Build history of the part. All positions in model axes, mm. A direction names the side the tool comes from. Round coordinates to 2 decimals unless told otherwise and drop trailing zeros. Write each loop counter-clockwise with the first axis right and the second up, starting at its lowest first coordinate (ties: lowest second). Pieces come first, ordered by that corner, then holes. Notation, with made-up numbers: (7.25, 53) -> (52.25, 53) arc R26 cw to (52.25, 67) -> close; hole circle Ø9 at (-15.75, 73.25). An arc over 180 degrees is marked (long way). Return JSON: item names as keys, results as strings.
from build123d import *

# Parameters (mm, degrees)
CUT_EXTRUDE_1_DEPTH = 3
FILLET_1_R          = 1
CHAMFER_1_SIZE      = 0.5


with BuildPart() as part:
    # 草图1 → 旋转1 (revolve)
    with BuildSketch(Plane.XY):
        Polygon((0, 0), (0, 5), (4.5, 5), (4.5, 3), (14.5, 3), (14.5, 2.5), (24.5, 2.5), (24.5, 0), align=None)
    revolve(axis=Axis((0, 0, 0), (1, 0, 0)))

    # 草图2 → 切除-拉伸1 (cut)
    with BuildSketch(Plane.ZY):
        Polygon((0, 1.732050808), (-1.5, 0.866025404), (-1.5, -0.866025404), (0, -1.732050808), (1.5, -0.866025404), (1.5, 0.866025404), align=None)
    extrude(amount=-CUT_EXTRUDE_1_DEPTH, mode=Mode.SUBTRACT)

    # 圆角1
    fillet_1_edges = [part.edges().sort_by_distance(p)[0] for p in [
        (0, -5, 0),
    ]]
    fillet(fillet_1_edges, radius=FILLET_1_R)

    # 倒角1
    chamfer_1_edges = [part.edges().sort_by_distance(p)[0] for p in [
        (24.5, -2.5, 0),
    ]]
    chamfer(chamfer_1_edges, length=CHAMFER_1_SIZE)


solid = part.part
Q1. 3-axis set-ups, long thin cutter, end or side, ignore diameter. For faces 4 (the cylindrical face through (19.32, -0.54, -2.44)), 5 (the flat face through (1.479, 1.293, 0.76)), 6 (the flat face through (0, -2, 0)): which of +Z, -Z, +X, -X, +Y, -Y reach the whole face in a straight line?
Verdict:
{"face 4": "+X", "face 5": "-X", "face 6": "+Z, -Z, -X, +Y, -Y"}
Q2. Saw through at C-C on x = 6.25. List the corners of the cut face in (y, z), then the cut area to 3 significant figures.
Verdict:
{"outline": "circle Ø6 at (0, 0)", "area": "28.3 mm²"}
Q3. Wall check: L1, parallel to Z at x = 6.5, y = 0; L2, parallel to X at y = 3, z = -2.5; L3, parallel to X at y = -2, z = -1.75. Give the ranges that are in metal, low to high.
Verdict:
{"L1": "z = -3 to 3", "L2": "x = 0 to 4.5", "L3": "x = 0 to 14.5"}
Q4. Pin check, flat tips, straight feed: pin 1 Ø5 at (x, z) = (7.5, -2) entering from -Y; pin 2 Ø5 at (x, y) = (12, -1.5) entering from +Z; pin 3 Ø2 at (y, z) = (1.5, 0.5) entering from -X; pin 4 Ø4 at (y, z) = (-3.5, 3.5) entering from +X. Stop position of each tip, or through.
Verdict:
{"pin 1": "stops at y = -3", "pin 2": "stops at z = 3", "pin 3": "stops at x = 0", "pin 4": "stops at x = 14.5"}
Q5. Saw through at B-B on y = 0. List the corners of the cut face in (x, z).
Verdict:
{"outline": "(0, -4) arc R1 ccw to (1, -5) -> (4.5, -5) -> (4.5, -3) -> (14.5, -3) -> (14.5, -2.5) -> (24, -2.5) -> (24.5, -2) -> (24.5, 2) -> (24, 2.5) -> (14.5, 2.5) -> (14.5, 3) -> (4.5, 3) -> (4.5, 5) -> (1, 5) arc R1 ccw to (0, 4) -> (0, 1.5) -> (3, 1.5) -> (3, -1.5) -> (0, -1.5) -> close"}
Q6. Two-plate mould, pull along Y, no slides. Class faces 1 (the flat face through (1, 0, -1.5)), 2 (the flat face through (24.5, 0, 0)), 3 (the cylindrical face through (2.77, -1.08, -4.88)): +Y half, -Y half, draft (parallel to the pull), parting line (faces both ways), or undercut.
Verdict:
{"face 1": "undercut", "face 2": "draft", "face 3": "parting line"}
Q7. Saw through at A-A on x = 2.5. List the corners of the cut face in (y, z), then the cut area to 3 significant figures.
Verdict:
{"outline": "circle Ø10 at (0, 0); hole (-1.73, 0) -> (-0.87, -1.5) -> (0.87, -1.5) -> (1.73, 0) -> (0.87, 1.5) -> (-0.87, 1.5) -> close", "area": "70.7 mm²"}
Q8. Saw through at D-D on x = 18.25. List the corners of the cut face in (y, z), then the cut area to 3 significant figures.
Verdict:
{"outline": "circle Ø5 at (0, 0)", "area": "19.6 mm²"}
